```python
from build123d import *

# Parameters (mm, degrees)
SKETCH_3_R                    = 2
CUT_EXTRUDE_1_DEPTH           = 4
SKETCH_4_R                    = 1
CUT_EXTRUDE_2_DEPTH           = 4
SKETCH_5_W                    = 2
SKETCH_5_H                    = 2
CUT_EXTRUDE_3_DEPTH           = 1.5
SKETCH_7_W                    = 2
SKETCH_7_H                    = 1.5
CUT_REVOLVE_1_ANGLE           = 45
CUT_REVOLVE_1_OTHER_WAY_ANGLE = 45


with BuildPart() as part:
    # Sketch 1 → Loft 1 section 0
    with BuildSketch(Plane(origin=(0, 0, 0), x_dir=(1, 0, 0), z_dir=(0, 1, 0))):
        with BuildLine():
            add(Edge.make_bspline(
                [(0, 0), (-0.026786257, 0.969360716), (0.61737566, 2.249301934), (1.974829337, 3.392775644), (2.993920842, 4.051952658), (4.355720519, 4.565101355), (5.990808256, 5.164346361), (8.017850303, 5.478919266), (10.008939201, 5.685410864), (12.675837367, 5.745020865), (16.011358195, 5.571319168), (20.019187774, 5.094065908), (23.99962122, 4.335399659), (28.002273256, 3.548249918), (31.989584978, 2.480873774), (36.034216793, 1.4621658), (38.689482894, 0.534654706), (39.98934, 0)],
                knots=[0, 0, 0, 0, 0.063515889, 0.095125078, 0.12262418, 0.147418569, 0.196010901, 0.243367076, 0.289416436, 0.335172983, 0.428593629, 0.521350126, 0.61548124, 0.710185536, 0.804793671, 0.902313957, 1, 1, 1, 1], degree=3))
            add(Edge.make_bspline(
                [(0, 0), (-0.026786257, -0.969360716), (0.61737566, -2.249301934), (1.974829337, -3.392775644), (2.993920842, -4.051952658), (4.355720519, -4.565101355), (5.990808256, -5.164346361), (8.017850303, -5.478919266), (10.008939201, -5.685410864), (12.675837367, -5.745020865), (16.011358195, -5.571319168), (20.019187774, -5.094065908), (23.99962122, -4.335399659), (28.002273256, -3.548249918), (31.989584978, -2.480873774), (36.034216793, -1.4621658), (38.689482894, -0.534654706), (39.98934, 0)],
                knots=[0, 0, 0, 0, 0.063515889, 0.095125078, 0.12262418, 0.147418569, 0.196010901, 0.243367076, 0.289416436, 0.335172983, 0.428593629, 0.521350126, 0.61548124, 0.710185536, 0.804793671, 0.902313957, 1, 1, 1, 1], degree=3))
        make_face()
    # Sketch 2 → Loft 1 section 1
    with BuildSketch(Plane(origin=(0, 13.15, 0), x_dir=(1, 0, 0), z_dir=(0, 1, 0))):
        with BuildLine():
            add(Edge.make_bspline(
                [(27.600495608, 0), (26.597023876, 0.239787804), (25.590303432, 0.450633429), (24.07845351, 0.751139895), (23.574236087, 0.848926057), (22.565707302, 1.043661503), (22.061334673, 1.140064965), (20.547046456, 1.418849109), (19.535800832, 1.589380729), (17.506159089, 1.866741534), (16.488154051, 1.977054776), (14.445960524, 2.142594028), (13.421688191, 2.197073085), (11.878361295, 2.217156944), (11.362851505, 2.21434148), (10.328296524, 2.177214316), (9.808955229, 2.140264674), (9.027129396, 2.059771774), (8.766490273, 2.029170171), (8.246673774, 1.962396763), (7.98718809, 1.926435537), (7.470450481, 1.84090371), (7.213172633, 1.791491042), (6.703084975, 1.665443783), (6.451257898, 1.58763007), (5.953139588, 1.420127607), (5.706204125, 1.330156877), (5.336512255, 1.193117575), (5.213271138, 1.147312759), (4.967522086, 1.054347625), (4.844966339, 1.007283734), (4.485806342, 0.850578332), (4.26912101, 0.704612862), (3.95354488, 0.468428314), (3.84988299, 0.385871664), (3.704605146, 0.253019135), (3.657777639, 0.207183214), (3.570159407, 0.109650945), (3.528407556, 0.058887646), (3.495024534, 0)],
                knots=[0, 0, 0, 0, 0.125, 0.125, 0.1875, 0.1875, 0.25, 0.25, 0.375, 0.375, 0.5, 0.5, 0.625, 0.625, 0.6875, 0.6875, 0.75, 0.75, 0.78125, 0.78125, 0.8125, 0.8125, 0.84375, 0.84375, 0.875, 0.875, 0.90625, 0.90625, 0.921875, 0.921875, 0.9375, 0.9375, 0.96875, 0.96875, 0.984375, 0.984375, 0.9921875, 0.9921875, 1, 1, 1, 1], degree=3))
            add(Edge.make_bspline(
                [(3.495024534, 0), (3.527836487, -0.057880281), (3.570196415, -0.109749182), (3.658869962, -0.20834136), (3.70652894, -0.254882194), (3.853181237, -0.388672418), (3.956462947, -0.470726548), (4.167794949, -0.628660052), (4.275587446, -0.704873243), (4.499789963, -0.846140938), (4.615390753, -0.907467588), (4.853487439, -1.01062304), (4.974416307, -1.056988781), (5.216688696, -1.148571028), (5.338066313, -1.193693034), (5.702321862, -1.328718991), (5.945643298, -1.417393741), (6.436562197, -1.582891985), (6.684094371, -1.659896431), (7.189108296, -1.786329481), (7.445644373, -1.836258275), (7.9566654, -1.921867633), (8.212450695, -1.957701806), (8.724233006, -2.023999353), (8.980232008, -2.054412341), (9.748649974, -2.134972616), (10.261536754, -2.173252617), (11.288759593, -2.213048165), (11.802997519, -2.217053051), (13.346857368, -2.199994887), (14.378737253, -2.146921583), (16.440497768, -1.981978581), (17.466695193, -1.87149656), (19.509569182, -1.59358314), (20.525655422, -1.422620707), (22.045907717, -1.142986252), (22.552073866, -1.046277871), (23.564078812, -0.850903032), (24.070010899, -0.752794594), (25.586627068, -0.45141053), (26.595958245, -0.240042446), (27.600495608, 0)],
                knots=[0, 0, 0, 0, 0.0078125, 0.0078125, 0.015625, 0.015625, 0.03125, 0.03125, 0.046875, 0.046875, 0.0625, 0.0625, 0.078125, 0.078125, 0.09375, 0.09375, 0.125, 0.125, 0.15625, 0.15625, 0.1875, 0.1875, 0.21875, 0.21875, 0.25, 0.25, 0.3125, 0.3125, 0.375, 0.375, 0.5, 0.5, 0.625, 0.625, 0.75, 0.75, 0.8125, 0.8125, 0.875, 0.875, 1, 1, 1, 1], degree=3))
        make_face()
    loft()

    # Sketch 3 → Cut-Extrude 1 (cut)
    with BuildSketch(Plane(origin=(0, 0, 0), x_dir=(1, 0, 0), z_dir=(0, 1, 0))):
        with Locations(Location((11.9968, 0, 0), (0, 0, 270))):
            Circle(SKETCH_3_R)
    extrude(amount=CUT_EXTRUDE_1_DEPTH, mode=Mode.SUBTRACT)

    # Sketch 4 → Cut-Extrude 2 (cut)
    with BuildSketch(Plane(origin=(0, 13.15, 0), x_dir=(1, 0, 0), z_dir=(0, 1, 0))):
        with Locations(Location((11.9968, 0, 0), (0, 0, 270))):
            Circle(SKETCH_4_R)
    extrude(amount=-CUT_EXTRUDE_2_DEPTH, mode=Mode.SUBTRACT)

    # Sketch 5 → Cut-Extrude 3 (cut)
    with BuildSketch(Plane.XZ):
        with Locations((17.75, 0)):
            Rectangle(SKETCH_5_W, SKETCH_5_H)
    extrude(amount=-CUT_EXTRUDE_3_DEPTH, mode=Mode.SUBTRACT)

    # Sketch 7 → Cut-Revolve 1 (revolve, cut)
    with BuildSketch(Plane.XY):
        with Locations((17.75, 0.75)):
            Rectangle(SKETCH_7_W, SKETCH_7_H)
    revolve(axis=Axis((11.9968, 4, 0), (0, -1, 0)), revolution_arc=CUT_REVOLVE_1_ANGLE, mode=Mode.SUBTRACT)

    # Sketch 7 → Cut-Revolve 1 other way (revolve, cut)
    with BuildSketch(Plane.XY):
        with Locations((17.75, 0.75)):
            Rectangle(SKETCH_7_W, SKETCH_7_H)
    revolve(axis=Axis((11.9968, 4, 0), (0, 1, 0)), revolution_arc=CUT_REVOLVE_1_OTHER_WAY_ANGLE, mode=Mode.SUBTRACT)


solid = part.part
```
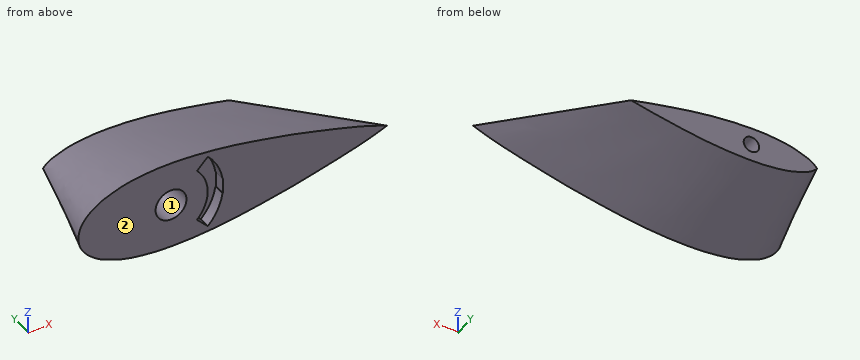
Geometry check sheet. Reference: the model listing, model coordinates, mm. Face numbers are marked on the shaded views. Give positions to 0.01 mm unless a question says otherwise; leave off trailing zeros.
1) Release check for a two-part mould opening along Z. For the marked faces 1 and 2 record: pulls with the +Z half, pulls with the -Z half, needs draft (parallel to the pull), parting line crosses it, or undercut.
2) Material ranges on L1, parallel to Z at x = 11.5, y = 9.75; L2, parallel to Z at x = 7.5, y = 3.5; L3, parallel to Z at x = 11, y = 8.75, recorded low to high.
3) Gauge pin test, flat ends, axial feed: pin 1 (4 mm diameter, centred on y = 8.5, z = -1.5, fed in from -X); pin 2 (1.6 mm diameter, centred on y = 1, z = 0.5, fed in from -X); pin 3 (5 mm diameter, centred on x = 22, y = 8, fed in from +Z). Record the tip position at first contact, or that the pin passes through.
Computed:
1. face 1: undercut
1. face 2: needs draft
2. L1: z = -3.12 to -0.87, 0.87 to 3.11
2. L2: z = -4.44 to 4.44
2. L3: z = -3.37 to 3.37
3. pin 1: stops at x = 1.9
3. pin 2: stops at x = 0.07
3. pin 3: stops at z = 3.31
